```python
from build123d import *

# Parameters (mm, degrees)
F0_W     = 50.8
F0_H     = 25.4
F1_DEPTH = 12.7
F2_W     = 12.7
F2_H     = 50.8
F3_DEPTH = 25.4
F4_R     = 7.62
F5_DEPTH = 53.34
F6_DEPTH = 25.4
F7_R     = 7.62
F8_DEPTH = 25.4


with BuildPart() as f1:
    # F0 (on Top) → F1 (new body)
    with BuildSketch(Plane.XY):
        Polygon((-27.004177, 22.899404), (-39.704177, 22.899404), (-39.704177, 10.199404), (11.095823, 10.199404), (11.095823, 22.899404), (-1.604177, 22.899404), align=None)
        Polygon((11.095823, -15.200596), (-39.704177, -15.200596), (-39.704177, -27.900596), (-27.004177, -27.900596), (-1.604177, -27.900596), (11.095823, -27.900596), align=None)
        with Locations((-14.304177, -2.500596)):
            Rectangle(F0_W, F0_H)
    extrude(amount=F1_DEPTH)

    # F2 (on face) → F3 (join)
    with BuildSketch(Plane.XY.offset(12.7)):
        with Locations((-33.354177, -2.500596)):
            Rectangle(F2_W, F2_H)
        with Locations((4.745823, -2.500596)):
            Rectangle(F2_W, F2_H)
    extrude(amount=F3_DEPTH)

    # F4 (on face) → F5 (cut)
    with BuildSketch(Plane(origin=(-39.704177, 0, 0), x_dir=(0, -1, 0), z_dir=(-1, 0, 0))):
        with BuildLine():
            ThreePointArc((-22.899404, 25.4), (2.500596, 38.014124), (27.900596, 25.4))
            Line((27.900596, 25.4), (27.900596, 38.1))
            Line((27.900596, 38.1), (-22.899404, 38.1))
            Line((-22.899404, 38.1), (-22.899404, 25.4))
        make_face()
        with Locations((2.500596, 25.4)):
            Circle(F4_R)
    extrude(amount=-F5_DEPTH, mode=Mode.SUBTRACT)

    # F0 (on Top) → F6 (join)
    with BuildSketch(Plane.XY):
        with Locations((-14.304177, -2.500596)):
            Rectangle(F0_W, F0_H)
    extrude(amount=-F6_DEPTH)

    # F7 (on face) → F8 (cut)
    with BuildSketch(Plane.XZ.offset(15.200596)):
        with Locations((-14.304177, -13.500606)):
            Circle(F7_R)
        with BuildLine():
            ThreePointArc((11.095823, -12.7), (-14.304177, -25.326352), (-39.704177, -12.7))
            Line((-39.704177, -12.7), (-39.704177, -25.4))
            Line((-39.704177, -25.4), (11.095823, -25.4))
            Line((11.095823, -25.4), (11.095823, -12.7))
        make_face()
    extrude(amount=-F8_DEPTH, mode=Mode.SUBTRACT)


solid = f1.part
```
Geometry check sheet. Reference: the model listing, model coordinates, mm. A direction names the side the tool comes from. Coordinates: 2 decimals unless noted, no trailing zeros. Write each loop counter-clockwise with the first axis right and the second up, starting at its lowest first coordinate (ties: lowest second). Pieces come first, ordered by that corner, then holes. Notation, with made-up numbers: M -35.75,13.5 L 2.25,13.5 A34 ccw 2.25,52.5 Z; hole C 59.25,57.5 d8. An arc over 180 degrees is marked long. Use one line per item in the form item = value. Start each with the question number.
1) Set-up check for faces 1 (the flat face through (-15, 10.199, -4)), 2 (the flat face through (-1.604, -3, 17)), 3 (the flat face through (-15, -15.201, -4)): record each of +Z, -Z, +X, -X, +Y, -Y from which the full face is reachable in a straight line by a thin tool's end or side.
2) Section check A-A on x = -32. Enter the section's corners in (y, z), and give its area (3 significant figures).
3) Thickness scan on probe 1 along X at (y, z) = (15, 13); probe 2 along Y at (x, z) = (-35, 25); probe 3 along Z at (x, y) = (-21, -21.5). Record the ranges inside material, lowest first. Write a range as from..to.
4) Go/stop test with flat-tipped pins: pin 1 Ø10 at (x, y) = (-17, 19) entering from -Z; pin 2 Ø10 at (x, z) = (-12.5, -16.5) entering from +Y; pin 3 Ø5 at (x, y) = (-12.5, -15) entering from +Z; pin 4 Ø7.5 at (x, z) = (-14, -16.5) entering from +Y. Record where each tip stops, or that it passes through.
5) Section check D-D on z = -4. Enter the section's corners in (x, y).
6) Section check C-C on y = 12.5. Enter the section's corners in (x, z).
7) Release check for a two-part mould opening along X. For faces 4 (the cylindrical face through (-13.893, -2.678, -25.324)), 5 (the flat face through (-14, -2, 12.7)), 6 (the flat face through (11.096, -3, 12)), 7 (the cylindrical face through (-33.44, -6.02, 18.64)) record: pulls with the +X half, pulls with the -X half, needs draft (parallel to the pull), parting line crosses it, or undercut.
8) Section check B-B on x = -10.5. Enter the section's corners in (y, z), and give its area (3 significant figures).
Responses:
q1.face_1 = -Z, +X, -X, +Y
q1.face_2 = +Z, +Y, -Y
q1.face_3 = -Z, +X, -X, -Y
q2.outline = M -27.9,0 L -15.2,0 L -15.2,-19.96 L 10.2,-19.96 L 10.2,0 L 22.9,0 L 22.9,25.4 A31.88 ccw -27.9,25.4 Z; hole C -2.5,25.4 d15.24
q2.area = 2,060 mm2
q3.probe_1 = -39.7..-27, -1.6..11.1
q3.probe_2 = -27.9..-10.11, 5.11..22.9
q3.probe_3 = 0..12.7
q4.pin_1 = 0
q4.pin_2 = 10.2
q4.pin_3 = 12.7
q4.pin_4 = through
q5.outline = M -39.7,-15.2 L 11.1,-15.2 L 11.1,10.2 L -39.7,10.2 Z
q6.outline = M -39.7,0 L 11.1,0 L 11.1,34.26 L -1.6,34.26 L -1.6,12.7 L -27,12.7 L -27,34.26 L -39.7,34.26 Z
q7.face_4 = parting line crosses it
q7.face_5 = undercut
q7.face_6 = pulls with the +X half
q7.face_7 = needs draft
q8.outline = M -27.9,0 L -15.2,0 L -15.2,-6.9 L 10.2,-6.9 L 10.2,0 L 22.9,0 L 22.9,12.7 L -27.9,12.7 Z; M -15.2,-25.1 L 10.2,-25.1 L 10.2,-20.1 L -15.2,-20.1 Z
q8.area = 947 mm2
